Verification items for the finished model (mm, model axes). Face numbers are marked on the shaded views. A direction names the side the tool comes from. Coordinates: 2 decimals unless noted, no trailing zeros. Loops run counter-clockwise (first coordinate to the right, second up) from the corner with the lowest first, then second, coordinate; pieces in that order, holes last. Notation, with made-up numbers: (-22, -3) - (-9, -3) arc R26 ccw to (-9, 28) - close; hole circle Ø10 at (-27.5, 63.5). An arc over 180 degrees is marked (long way). One line per item, written item: value. Start each with the question number.
(1) Set-up check for the marked faces 1, 2, 3 and 4: record each of +Z, -Z, +X, -X, +Y, -Y from which the full face is reachable in a straight line by a thin tool's end or side.
(2) Section check A-A (y = 110). Record the boundary of the cut face in (x, z) (3 decimals), plus the area to 3 significant figures.
(3) Section check B-B (y = 0). Record the boundary of the cut face in (x, z) (3 decimals), plus the area to 3 significant figures.
(4) Section check C-C (x = 66). Record the boundary of the cut face in (y, z) (3 decimals).
(5) Thickness scan on probe 1 along Z at (x, y) = (58, 97.5) (3 decimals); probe 2 along Z at (x, y) = (-23, 30); probe 3 along Y at (x, z) = (36, -45). Record the ranges inside material, lowest first. Write a range as [from, to].
(6) Section check D-D (z = -14.5). Record the boundary of the cut face in (x, y).
(7) Gauge pin test, flat ends, axial feed: P1, Ø20.5, axis at x = -60, y = 87, coming from the -Z side; P2, Ø7, axis at x = -73.5, y = -13, coming from the +Z side; P3, Ø3.5, axis at y = 29, z = 1.5, coming from the -X side. Record the tip position at first contact, or that the pin passes through.
```python
from build123d import *

# Parameters (mm, degrees)
F0_R     = 76.2
F1_DEPTH = 50.8
F2_W     = 25.4
F2_H     = 254
F3_DEPTH = 3.175


with BuildPart() as f1:
    # F0 (on Top) → F1 (new body)
    with BuildSketch(Plane.XY):
        Circle(F0_R)
    extrude(amount=-F1_DEPTH)

    # F2 (on Top) → F3 (join)
    with BuildSketch(Plane.XY):
        with Locations((-57.15, 50.8)):
            Rectangle(F2_W, F2_H)
        with Locations((57.15, 50.8)):
            Rectangle(F2_W, F2_H)
    extrude(amount=F3_DEPTH)


solid = f1.part
```
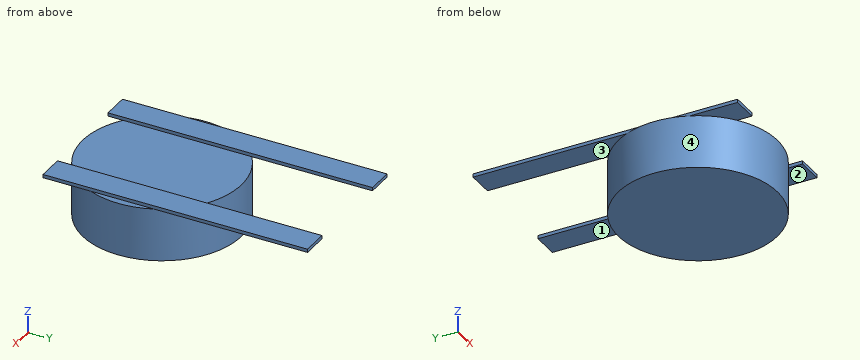
Responses:
1. face 1: -Z, +X, +Y
1. face 2: -Z, +X, -Y
1. face 3: -Z, -X, +Y
1. face 4: -Z
2. outline: (-69.85, 0) - (-44.45, 0) - (-44.45, 3.175) - (-69.85, 3.175) - close; (44.45, 0) - (69.85, 0) - (69.85, 3.175) - (44.45, 3.175) - close
2. area: 161 mm²
3. outline: (-76.2, -50.8) - (76.2, -50.8) - (76.2, 0) - (69.85, 0) - (69.85, 3.175) - (44.45, 3.175) - (44.45, 0) - (-44.45, 0) - (-44.45, 3.175) - (-69.85, 3.175) - (-69.85, 0) - (-76.2, 0) - close
3. area: 7,900 mm²
4. outline: (-76.2, 0) - (-38.085, 0) - (-38.085, -50.8) - (38.085, -50.8) - (38.085, 0) - (177.8, 0) - (177.8, 3.175) - (-76.2, 3.175) - close
5. probe 1: z = [0, 3.175]
5. probe 2: z = [-50.8, 0]
5. probe 3: y = [-67.16, 67.16]
6. outline: circle Ø152.4 at (0, 0)
7. P1: stops at z = 0
7. P2: stops at z = 0
7. P3: stops at x = -70.83
